Design review of the part built by this model. Coordinates are the model's own, in mm. A direction names the side the tool comes from. Give positions to 0.01 mm unless a question says otherwise; leave off trailing zeros. Loops run counter-clockwise (first coordinate to the right, second up) from the corner with the lowest first, then second, coordinate; pieces in that order, holes last. Notation, with made-up numbers: M 5.25,5 L 62.25,5 A21 cw 62.25,33 Z; hole C 14.25,-14.75 d6. An arc over 180 degrees is marked long. Use one line per item in the form item = value. Start each with the question number.
from build123d import *

# Parameters (mm, degrees)
EXTRUDE_1_DEPTH          = 2
SKETCH_3_R               = 1.4
CUT_EXTRUDE_2_DEPTH      = 1
SKETCH_4_R               = 0.8
CUT_EXTRUDE_3_DEPTH      = 7
FILLET_1_R               = 1
EXTRUDE_2_DEPTH          = 1.79
EXTRUDE_3_DEPTH          = 6.8
CUT_EXTRUDE_4_DEPTH      = 2
CUT_EXTRUDE_5_DEPTH      = 9
CUT_EXTRUDE_5_DEPTH_BACK = 5
SKETCH_8_R               = 28.905330341
FILLET_2_R               = 1


with BuildPart() as part:
    # Sketch 1 → Extrude 1 (new body)
    with BuildSketch(Plane(origin=(0, 0, 0), x_dir=(1, 0, 0), z_dir=(0, 1, 0))):
        with BuildLine():
            Line((50.296518896, 15.038773117), (51.995638969, 15.038535751))
            Line((51.995638969, 15.038535751), (51.99484152, 5.380301086))
            Line((51.99484152, 5.380301086), (50.29420013, 5.380011427))
            Line((50.29420013, 5.380011427), (50.293979101, 3.999471495))
            ThreePointArc((50.293979101, 3.999471495), (49.619955043, 2.373282378), (47.993458708, 1.700000008))
            Line((47.993458708, 1.700000008), (3.993570964, 1.700000008))
            ThreePointArc((3.993570964, 1.700000008), (2.367381847, 2.374024066), (1.694099477, 4.000520401))
            Line((1.694099477, 4.000520401), (1.718930657, 16.432494262))
            ThreePointArc((1.718930657, 16.432494262), (2.392954716, 18.058683379), (4.01945105, 18.731965749))
            Line((4.01945105, 18.731965749), (47.997365049, 18.71993116))
            ThreePointArc((47.997365049, 18.71993116), (49.623554167, 18.045907101), (50.296836537, 16.419410767))
            Line((50.296836537, 16.419410767), (50.296518896, 15.038773117))
        make_face()
    extrude(amount=EXTRUDE_1_DEPTH)

    # Sketch 3 → Cut-Extrude 2 (cut)
    with BuildSketch(Plane(origin=(0, 0, 0), x_dir=(1, 0, 0), z_dir=(0, 1, 0))):
        with Locations(Location((4.986997661, 16.769823075, 0), (0, 0, 270))):
            Circle(SKETCH_3_R)
        with Locations(Location((4.984007822, 3.657835416, 0), (0, 0, 270))):
            Circle(SKETCH_3_R)
        with Locations(Location((44.986916621, 16.760702161, 0), (0, 0, 270))):
            Circle(SKETCH_3_R)
        with Locations(Location((44.983926782, 3.648714502, 0), (0, 0, 270))):
            Circle(SKETCH_3_R)
    extrude(amount=CUT_EXTRUDE_2_DEPTH, mode=Mode.SUBTRACT)

    # Sketch 4 → Cut-Extrude 3 (cut)
    with BuildSketch(Plane(origin=(0, 2, 0), x_dir=(1, 0, 0), z_dir=(0, 1, 0))):
        with Locations(Location((44.983926782, 3.648714502, 0), (0, 0, 270))):
            Circle(SKETCH_4_R)
        with Locations(Location((44.986916621, 16.760702161, 0), (0, 0, 270))):
            Circle(SKETCH_4_R)
        with Locations(Location((4.984007822, 3.657835416, 0), (0, 0, 270))):
            Circle(SKETCH_4_R)
        with Locations(Location((4.986997661, 16.769823075, 0), (0, 0, 270))):
            Circle(SKETCH_4_R)
    extrude(amount=-CUT_EXTRUDE_3_DEPTH, mode=Mode.SUBTRACT)

    # Fillet 1
    fillet_1_edges = [part.edges().sort_by_distance(p)[0] for p in [
        (51.995240244, 0, -10.209418418),
    ]]
    fillet(fillet_1_edges, radius=FILLET_1_R)

    # Sketch 5 → Extrude 2 (add)
    with BuildSketch(Plane(origin=(0, 2, 0), x_dir=(1, 0, 0), z_dir=(0, 1, 0))):
        Polygon((1.715661177, 14.795597045), (5.715661177, 14.795597045), (5.715661177, 5.660468281), (1.697415134, 5.660536688), align=None)
    extrude(amount=EXTRUDE_2_DEPTH)


with BuildPart() as extrude_3_tool:
    # Sketch 6 → Extrude 3 (new body)
    with BuildSketch(Plane(origin=(0, 0, 0), x_dir=(1, 0, 0), z_dir=(0, 1, 0))):
        Polygon((35.908795328, 20.423234707), (35.908407688, 18.723234749), (16.108408411, 18.72866216), (16.108796051, 20.428662118), align=None)
    extrude(amount=EXTRUDE_3_DEPTH)


with BuildPart() as part_1:
    add(part.part)


with BuildPart() as part_2:
    # Extrude 3: joined with extrude_3_tool
    add(part_1.part.fuse(extrude_3_tool.part, tol=0.00001))

    # Sketch 7 → Cut-Extrude 4 (cut)
    with BuildSketch(Plane(origin=(0, 6.8, 0), x_dir=(1, 0, 0), z_dir=(0, 1, 0))):
        with BuildLine():
            Line((20.454642354, 18.427468236), (32.137878346, 18.424271109))
            ThreePointArc((32.137878346, 18.424271109), (26.297078845, 21.416891462), (20.454642354, 18.427468236))
        make_face()
    extrude(amount=-CUT_EXTRUDE_4_DEPTH, mode=Mode.SUBTRACT)

    # Sketch 8 → Cut-Extrude 5 (cut, two sides: drawn at the far end of the back side and taken through both)
    with BuildSketch(Plane(origin=(0, 2, 0), x_dir=(1, 0, 0), z_dir=(0, 1, 0)).offset(-CUT_EXTRUDE_5_DEPTH_BACK)):
        with Locations((26.015215658, 48.580825692)):
            Circle(SKETCH_8_R)
    extrude(amount=CUT_EXTRUDE_5_DEPTH + CUT_EXTRUDE_5_DEPTH_BACK, mode=Mode.SUBTRACT)

    # Fillet 2
    fillet_2_edges = [part_2.edges().sort_by_distance(p)[0] for p in [
        (34.230033191, 0, -20.423694875),
        (17.786260576, 0, -20.428202305),
        (26.00729237, 0, -19.675496437),
    ]]
    fillet(fillet_2_edges, radius=FILLET_2_R)


solid = part_2.part
Q1. The part is to be moulded in two halves that separate along Z. For faces 3 (the flat face through (4, 3.79, -10)), 4 (the cylindrical face through (17.81, 0.29, -20.13)), 5 (the cylindrical face through (4.274, 1.507, -3.289)), say which applies: pulls with the +Z half, pulls with the -Z half, needs draft (parallel to the pull), parting line crosses it, or undercut.
Q2. Take a section at A-A on z = -3.5. Give the boundary of the cut face in (x, y).
Q3. Clearance check with flat-ended pins moving along their axes: pin 1 Ø1.9 at (y, z) = (3, -20) entering from +X; pin 2 Ø1.6 at (x, y) = (45, 1) entering from -Z; pin 3 Ø0.9 at (x, y) = (3, 3) entering from +Z; pin 4 Ø0.8 at (x, z) = (45, -16.5) entering from -Y. State where each tip first meets the part, or that it passes through.
Q4. Take a section at B-B on y = 0.5. Give the boundary of the cut face in (x, z), plus the area to 3 significant figures.
Q5. Take a section at D-D on x = 14.5. Give the boundary of the cut face in (y, z), plus the area to 3 significant figures.
Q6. For faces 1 (the cylindrical face through (4.451, 0.493, -15.477)), 2 (the flat face through (34, 6.8, -20)), list the 3-axis set-ups (+Z, -Z, +X, -X, +Y, -Y) from which the entire face can be reached by the end or side of a thin tool; tool diameter is ignored.
Q7. Wall thickness on probe 1 along X at (y, z) = (1.5, -4.25); probe 2 along Y at (x, z) = (36.5, -8.5); probe 3 along Z at (x, y) = (30, 1): over which ranges is each line inside the solid? List them lowest first.
Q8. Take a section at C-C on x = 40.5. Give the boundary of the cut face in (y, z), plus the area to 3 significant figures.
Response values:
q1.face_3 = needs draft
q1.face_4 = pulls with the -Z half
q1.face_5 = undercut
q2.outline = M 1.75,0 L 3.59,0 L 3.59,1 L 4.2,1 L 4.2,2 L 1.75,2 Z; M 5.77,1 L 6.38,1 L 6.38,0 L 43.59,0 L 43.59,1 L 44.2,1 L 44.2,2 L 5.77,2 Z; M 45.77,1 L 46.38,1 L 46.38,0 L 50.24,0 L 50.24,2 L 45.77,2 Z
q3.pin_1 = 35.91
q3.pin_2 = -18.72
q3.pin_3 = -5.66
q3.pin_4 = through
q4.outline = M 1.69,-4 L 1.72,-16.43 A2.3 ccw 4.02,-18.73 L 16.11,-18.73 L 16.11,-20.29 L 19.45,-20.29 A29.04 cw 32.57,-20.29 L 35.91,-20.29 L 35.91,-18.72 L 48,-18.72 A2.3 ccw 50.3,-16.42 L 50.3,-15.04 L 51.86,-15.04 L 51.86,-5.38 L 50.29,-5.38 L 50.29,-4 A2.3 ccw 47.99,-1.7 L 3.99,-1.7 A2.3 ccw Z; hole C 4.98,-3.66 d2.8; hole C 4.99,-16.77 d2.8; hole C 44.98,-3.65 d2.8; hole C 44.99,-16.76 d2.8
q4.area = 838 mm^2
q5.outline = M 0,-18.73 L 2,-18.73 L 2,-1.7 L 0,-1.7 Z
q5.area = 34.1 mm^2
q6.face_1 = -Y
q6.face_2 = +Z, -Z, +X, -X, +Y
q7.probe_1 = 1.69 to 4.45, 5.52 to 44.46, 45.51 to 50.29
q7.probe_2 = 0 to 2
q7.probe_3 = -19.95 to -1.7
q8.outline = M 0,-18.72 L 2,-18.72 L 2,-1.7 L 0,-1.7 Z
q8.area = 34.0 mm^2
